Could you check a few things on this model? Use its own coordinates, in mm. Coordinates: 2 decimals unless noted, no trailing zeros. Write each loop counter-clockwise with the first axis right and the second up, starting at its lowest first coordinate (ties: lowest second). Pieces come first, ordered by that corner, then holes.
```python
from build123d import *

# Parameters (mm, degrees)
F1_W     = 50.8
F1_H     = 50.8
F2_DEPTH = 1778
F3_R     = 12.7
F4_T     = -6.35


with BuildPart() as f2:
    # F1 (on face) → F2 (new body)
    with BuildSketch(Plane.XZ):
        with Locations((25.4, 25.4)):
            Rectangle(F1_W, F1_H)
    extrude(amount=F2_DEPTH)

    # F3
    f3_edges = [f2.edges().sort_by_distance(p)[0] for p in [
        (0, -889, 50.8),
        (0, -889, 0),
        (50.8, -889, 50.8),
        (50.8, -889, 0),
    ]]
    fillet(f3_edges, radius=F3_R)

    # F4
    f4_openings = [f2.faces().sort_by_distance(p)[0] for p in [
        (25.4, -1778, 25.4),
    ]]
    offset(amount=F4_T, openings=f4_openings)


solid = f2.part
```
1. I want a section at C-C on z = 23. Please give me the cut outline in (x, y).
Verdict:
outline: (0, -1778) - (6.35, -1778) - (6.35, -6.35) - (44.45, -6.35) - (44.45, -1778) - (50.8, -1778) - (50.8, 0) - (0, 0) - close
2. I want a section at B-B on y = -1428. Please give me the cut outline in (x, z).
Verdict:
outline: (0, 12.7) arc R12.7 ccw to (12.7, 0) - (38.1, 0) arc R12.7 ccw to (50.8, 12.7) - (50.8, 38.1) arc R12.7 ccw to (38.1, 50.8) - (12.7, 50.8) arc R12.7 ccw to (0, 38.1) - close; hole (6.35, 12.7) arc R6.35 ccw to (12.7, 6.35) - (38.1, 6.35) arc R6.35 ccw to (44.45, 12.7) - (44.45, 38.1) arc R6.35 ccw to (38.1, 44.45) - (12.7, 44.45) arc R6.35 ccw to (6.35, 38.1) - close
3. Please list where this line runs through material, in increasing order: line 1 along X through (y, z) = (-390, 17).
Verdict:
line 1: x = 0 to 6.35, 44.45 to 50.8
4. For pin 1 (8 mm diameter, centred on x = 44.5, y = -657.5, fed in from -Z); pin 2 (5 mm diameter, centred on x = 35.5, z = 35.5, fed in from -Y); pin 3 (1.5 mm diameter, centred on x = 44.5, y = -587, fed in from +Z), each with a flat end and sliding along its axis, tell me the tip position at first contact or that it passes through.
Verdict:
pin 1: stops at z = 0.23
pin 2: stops at y = -6.35
pin 3: stops at z = 49.47
5. If we mould it in two halves opening along Z, with no side actions, what happens to faces 1 (the face through (46, -1778, 27)), 2 (the face through (25, -6.35, 26))? For each: pulls with the +Z half, pulls with the -Z half, needs draft (parallel to the pull), parting line crosses it, or undercut.
Verdict:
face 1: needs draft
face 2: undercut
6. I want a section at A-A on x = 27.5. Please give me the cut outline in (y, z), plus the area to 3 significant figures.
Verdict:
outline: (-1778, 0) - (0, 0) - (0, 50.8) - (-1778, 50.8) - (-1778, 44.45) - (-6.35, 44.45) - (-6.35, 6.35) - (-1778, 6.35) - close
area: 22,800 mm2
